from build123d import *

# Parameters (mm, degrees)
F0_W      = 80
F0_H      = 100
F1_DEPTH  = 34
F2_W      = 29
F2_H      = 9
F2_W_2    = 36
F2_H_2    = 16.5
F4_DEPTH  = 31
F5_DEPTH  = 85
F3_W      = 2
F3_H      = 10.5
F6_DEPTH  = 80
F2_W_3    = 24
F2_H_3    = 12.5
F2_R      = 0.5
F7_DEPTH  = 37
F8_DEPTH  = 31
F2_W_4    = 25
F2_H_4    = 5
F9_DEPTH  = 30
F10_DEPTH = 17
F12_DEPTH = 15
F13_DEPTH = 6
F14_DEPTH = 20


with BuildPart() as f1:
    # F0 (on Top) → F1 (new body)
    with BuildSketch(Plane.XY):
        with Locations((40, 50)):
            Rectangle(F0_W, F0_H)
    extrude(amount=F1_DEPTH)

    # F2 (on face) → F4 (cut)
    with BuildSketch(Plane.XY.offset(34)):
        Polygon((57.25, 15), (57.25, 100), (0, 100), (0, 2), (80, 2), (80, 100), (69.75, 100), (69.75, 15), align=None)
        with Locations((63.5, 7.5)):
            Rectangle(F2_W, F2_H, mode=Mode.SUBTRACT)
        with Locations((21, 50.25)):
            Rectangle(F2_W_2, F2_H_2, mode=Mode.SUBTRACT)
    extrude(amount=-F4_DEPTH, mode=Mode.SUBTRACT)

    # F3 (on face) → F5 (cut)
    with BuildSketch(Plane(origin=(0, 100, 0), x_dir=(-1, 0, 0), z_dir=(0, 1, 0))):
        Polygon((-67.75, 11.75), (-67.75, 9.75), (-59.25, 9.75), (-59.25, 11.75), (-59.25, 22.25), (-59.25, 24.25), (-67.75, 24.25), (-67.75, 22.25), align=None)
    extrude(amount=-F5_DEPTH, mode=Mode.SUBTRACT)

    # F3 (on face) → F6 (cut)
    with BuildSketch(Plane(origin=(0, 100, 0), x_dir=(-1, 0, 0), z_dir=(0, 1, 0))):
        with Locations((-58.25, 17)):
            Rectangle(F3_W, F3_H)
        with Locations((-68.75, 17)):
            Rectangle(F3_W, F3_H)
    extrude(amount=-F6_DEPTH, mode=Mode.SUBTRACT)

    # F2 (on face) → F7 (cut)
    with BuildSketch(Plane.XY.offset(34)):
        with Locations((21, 50.25)):
            Rectangle(F2_W_3, F2_H_3)
        with Locations((6.5, 50)):
            Circle(F2_R)
        with Locations((35.5, 50)):
            Circle(F2_R)
    extrude(amount=-F7_DEPTH, mode=Mode.SUBTRACT)

    # F2 (on face) → F8 (cut)
    with BuildSketch(Plane.XY.offset(34)):
        with Locations((21, 50.25)):
            Rectangle(F2_W_2, F2_H_2)
        with Locations((6.5, 50)):
            Circle(F2_R, mode=Mode.SUBTRACT)
        with Locations((21, 50.25)):
            Rectangle(F2_W_3, F2_H_3, mode=Mode.SUBTRACT)
        with Locations((35.5, 50)):
            Circle(F2_R, mode=Mode.SUBTRACT)
    extrude(amount=-F8_DEPTH, mode=Mode.SUBTRACT)

    # F2 (on face) → F9 (cut)
    with BuildSketch(Plane.XY.offset(34)):
        with Locations((63.5, 7.5)):
            Rectangle(F2_W_4, F2_H_4)
    extrude(amount=-F9_DEPTH, mode=Mode.SUBTRACT)

    # F2 (on face) → F10 (cut)
    with BuildSketch(Plane.XY.offset(34)):
        with Locations((63.5, 7.5)):
            Rectangle(F2_W, F2_H)
        with Locations((63.5, 7.5)):
            Rectangle(F2_W_4, F2_H_4, mode=Mode.SUBTRACT)
    extrude(amount=-F10_DEPTH, mode=Mode.SUBTRACT)

    # F11 (on face) → F12 (cut)
    with BuildSketch(Plane(origin=(0, 12, 0), x_dir=(-1, 0, 0), z_dir=(0, 1, 0))):
        with BuildLine():
            ThreePointArc((-71.4303621394, 17), (-63.5, 9.0696378606), (-55.5696378606, 17))
            Line((-55.5696378606, 17), (-71.4303621394, 17))
        make_face()
    extrude(amount=-F12_DEPTH, mode=Mode.SUBTRACT)

    # F13 (cut): a face of the model
    f13_faces = [f1.faces().sort_by_distance(p)[0] for p in [
        (63.5, 57.5, 34),
    ]]
    extrude(f13_faces, amount=-F13_DEPTH, mode=Mode.SUBTRACT)

    # F14 (cut): a face of the model
    f14_faces = [f1.faces().sort_by_distance(p)[0] for p in [
        (40, 1, 34),
    ]]
    extrude(f14_faces, amount=-F14_DEPTH, mode=Mode.SUBTRACT)


solid = f1.part
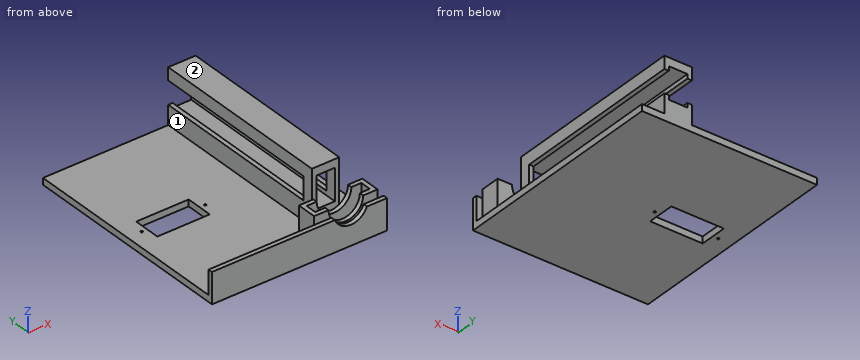
Could you check a few things on this model? Use its own coordinates, in mm. Face numbers are marked on the shaded views. A direction names the side the tool comes from. Round coordinates to 2 decimals unless told otherwise and drop trailing zeros. Write each loop counter-clockwise with the first axis right and the second up, starting at its lowest first coordinate (ties: lowest second). Pieces come first, ordered by that corner, then holes. Notation, with made-up numbers: (76, -18.5) - (94, -18.5) arc R28 ccw to (94, 19.5) - close; hole circle Ø10 at (77.25, -32). An arc over 180 degrees is marked (long way). Use a Markdown table: item, result.
Q1. I want a section at D-D (z = 20.25). List the corners of the cut face in (x, y) for me, plus the area to 3 significant figures.
Output values:
| item | result |
|---|---|
| outline | (57.25, 15) - (59.25, 15) - (59.25, 20) - (57.25, 20) - close; (67.75, 15) - (69.75, 15) - (69.75, 20) - (67.75, 20) - close |
| area | 20.0 mm2 |
Q2. I want a section at A-A (z = 6.5). List the corners of the cut face in (x, y) for me, plus the area to 3 significant figures.
Output values:
| item | result |
|---|---|
| outline | (0, 0) - (80, 0) - (80, 2) - (0, 2) - close; (49, 3) - (78, 3) - (78, 12) - (49, 12) - close; (57.25, 15) - (69.75, 15) - (69.75, 100) - (57.25, 100) - close; hole (51, 5) - (76, 5) - (76, 10) - (51, 10) - close |
| area | 1,360 mm2 |
Q3. Please list where these lines run through material, in increasing order: L1, parallel to Y at x = 58, z = 7.5; L2, parallel to X at y = 50, z = 1.55; L3, parallel to Z at x = 67, y = 69.5.
Output values:
| item | result |
|---|---|
| L1 | 0 to 2, 3 to 5, 10 to 12, 15 to 100 |
| L2 | 0 to 6, 7 to 9, 33 to 35, 36 to 80 |
| L3 | 0 to 9.75, 24.25 to 28 |
Q4. I want a section at B-B (x = 28.5). List the corners of the cut face in (y, z) for me.
Output values:
| item | result |
|---|---|
| outline | (0, 0) - (44, 0) - (44, 3) - (2, 3) - (2, 14) - (0, 14) - close; (56.5, 0) - (100, 0) - (100, 3) - (56.5, 3) - close |
Q5. I want a section at C-C (y = 30.5). List the corners of the cut face in (x, z) for me.
Output values:
| item | result |
|---|---|
| outline | (0, 0) - (80, 0) - (80, 3) - (69.75, 3) - (69.75, 11.75) - (67.75, 11.75) - (67.75, 9.75) - (59.25, 9.75) - (59.25, 11.75) - (57.25, 11.75) - (57.25, 3) - (0, 3) - close; (57.25, 22.25) - (59.25, 22.25) - (59.25, 24.25) - (67.75, 24.25) - (67.75, 22.25) - (69.75, 22.25) - (69.75, 28) - (57.25, 28) - close |
Q6. For the marked faces 1 and 2, which set-ups out of +Z, -Z, +X, -X, +Y, -Y let a thin tool reach every point of the face, with its end or its side?
Output values:
| item | result |
|---|---|
| face 1 | +Z, -X, +Y |
| face 2 | +Z, +X, -X, +Y, -Y |
Q7. For pin 1 (12 mm diameter, centred on x = 20.5, z = 7, fed in from +Y); pin 2 (10 mm diameter, centred on x = 61, z = 17, fed in from -Y); pin 3 (4 mm diameter, centred on y = 85, z = 23.5, fed in from +X); pin 4 (1.6 mm diameter, centred on x = 69, z = 16.5, fed in from +Y), each with a flat end and sliding along its axis, tell me the tip position at first contact or that it passes through.
Output values:
| item | result |
|---|---|
| pin 1 | y = 100 |
| pin 2 | y = 15 |
| pin 3 | x = 69.75 |
| pin 4 | y = 20 |
